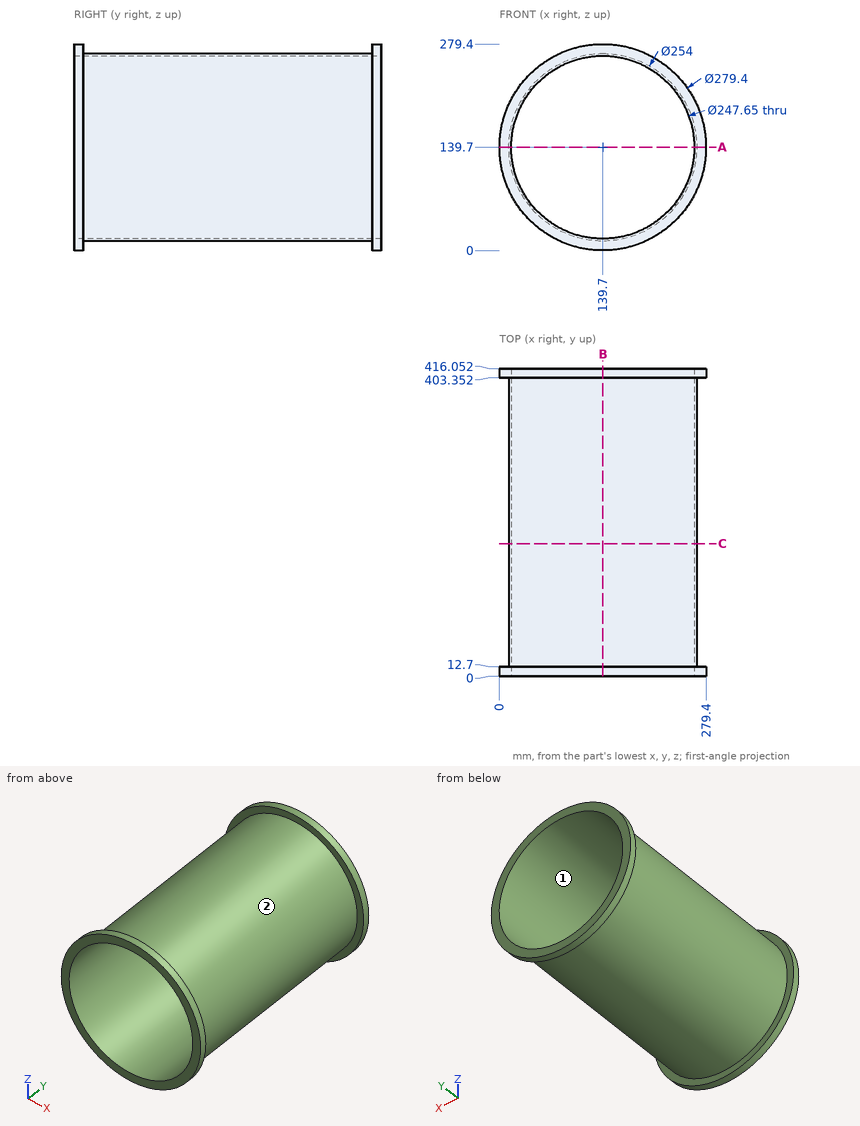
For this review, use the dimensioned drawing (mm, ordinates from the lowest corner) and the shaded views. Give positions to 0.01 mm unless a question says otherwise; leave off trailing zeros. Loops run counter-clockwise (first coordinate to the right, second up) from the corner with the lowest first, then second, coordinate; pieces in that order, holes last. Notation, with made-up numbers: (48, 3.25) -> (55, 3.25) arc R34 ccw to (55, 33.25) -> close; hole circle Ø2 at (23.25, -29.5). An arc over 180 degrees is marked (long way). Use CSV: the item, a comma, the result in double quotes.
1. Consider section A-A, the plane z = 139.7. Write out the cut boundary in (x, y) (3 decimals), then the cut area to 3 significant figures.
Result:
outline,"(0, 0) -> (15.875, 0) -> (15.875, 416.052) -> (0, 416.052) -> (0, 403.352) -> (12.7, 403.352) -> (12.7, 12.7) -> (0, 12.7) -> close; (263.525, 0) -> (279.4, 0) -> (279.4, 12.7) -> (266.7, 12.7) -> (266.7, 403.352) -> (279.4, 403.352) -> (279.4, 416.052) -> (263.525, 416.052) -> close"
area,"3,290 mm²"
2. To check wall thickness, follow probe 1 along X at (y, z) = (208.5, 139.7) (3 decimals); probe 2 along Y at (x, z) = (44.5, 40); probe 3 along Z at (x, y) = (139, 288). State the ranges of each line that lie inside material, in increasing order. Write a range as from..to.
Result:
probe 1,"x = 12.7..15.875, 263.525..266.7"
probe 2,"y = 0..12.7, 403.35..416.05"
probe 3,"z = 12.7..15.88, 263.52..266.7"
3. For P1, Ø10, axis at x = 175.5, y = 150, coming from the -Z side; P2, Ø1.5, axis at y = 72, z = 206, coming from the -X side; P3, Ø6, axis at x = 229.5, y = 322, coming from the +Z side, all flat-tipped, find the tip position at first contact; note any pin that passes through.
Result:
P1,"stops at z = 16.49"
P2,"stops at x = 30.92"
P3,"stops at z = 232.41"
4. Consider section C-C, the plane y = 179. Write out the cut boundary in (x, z) (3 decimals), then the cut area to 3 significant figures.
Result:
outline,"circle Ø254 at (139.7, 139.7); hole circle Ø247.65 at (139.7, 139.7)"
area,"2,500 mm²"
5. The part is to be moulded in two halves that separate along Z. For the marked faces 1 and 2, say which applies: +Z half, -Z half, draft (parallel to the pull), parting line (faces both ways), or undercut.
Result:
face 1,"undercut"
face 2,"parting line"
6. Consider section B-B, the plane x = 139.7. Write out the cut boundary in (y, z) (3 decimals).
Result:
outline,"(0, 0) -> (12.7, 0) -> (12.7, 12.7) -> (403.352, 12.7) -> (403.352, 0) -> (416.052, 0) -> (416.052, 15.875) -> (0, 15.875) -> close; (0, 263.525) -> (416.052, 263.525) -> (416.052, 279.4) -> (403.352, 279.4) -> (403.352, 266.7) -> (12.7, 266.7) -> (12.7, 279.4) -> (0, 279.4) -> close"
